```python
from build123d import *

# Parameters (mm, degrees)
CUT_EXTRUDE1_DEPTH = 46.95650117230423
FILLET1_R          = 10


with BuildPart() as part:
    # Sketch1 → Revolve1 (revolve)
    with BuildSketch(Plane.XY, mode=Mode.PRIVATE) as revolve1_sk:
        with BuildLine():
            Line((-20, 4.7625), (-20, 14.5))
            Line((-20, 14.5), (-15.328636266651278, 14.5))
            ThreePointArc((-15.328636266651278, 14.5), (1.5695766523512105, 11), (18.08622279664887, 16))
            Line((18.08622279664887, 16), (20, 16))
            Line((20, 16), (20, 4.7625))
            Line((20, 4.7625), (16.825, 4.7625))
            Line((16.825, 4.7625), (16.825, 3.96875))
            Line((16.825, 3.96875), (-16.825, 3.96875))
            Line((-16.825, 3.96875), (-16.825, 4.7625))
            Line((-16.825, 4.7625), (-20, 4.7625))
        make_face()
    revolve(revolve1_sk.sketch.rotate(Axis((-20, 0, 0), (1, 0, 0)), 90), axis=Axis((-20, 0, 0), (1, 0, 0)))

    # Sketch2 → Cut-Extrude1 (cut, through all)
    with BuildSketch(Plane(origin=(20, 0, 0), x_dir=(0, 0, -1), z_dir=(1, 0, 0))):
        Polygon((-0.9875675416844027, 5.918167820416334), (0, 8), (0.9875675416844045, 5.918167820416334), (2.5975957536374685, 7.56653793360508), (2.855684358222442, 5.276842507238936), (4.913701701517343, 6.313124075171151), (4.414343464038791, 4.06368942975445), (6.69733182610023, 4.375585264979419), (5.494639959930347, 2.4101725479178207), (7.7552021275146465, 1.9638838971263979), (5.979506958040023, 0.4954760728339973), (7.972675944053363, -0.6606347637786543), (5.8164015956359885, -1.47291292284479), (7.326186613240466, -3.2135633972237505), (5.022998869575178, -3.2816889487345575), (5.885791285385062, -5.418252573005925), (3.685276276138015, -4.7348430563783594), (3.807579144296598, -7.035790009651912), (1.948196815228109, -5.674903450203807), (1.3167567222458805, -7.890890427221779), (8.4e-15, -6), (-1.3167567222458623, -7.8908904272217795), (-1.9481968152280928, -5.674903450203809), (-3.80757914429658, -7.035790009651914), (-3.685276276137998, -4.7348430563783666), (-5.885791285385044, -5.418252573005935), (-5.022998869575163, -3.2816889487345664), (-7.326186613240452, -3.213563397223763), (-5.816401595635977, -1.4729129228448008), (-7.9726759440533534, -0.6606347637786659), (-5.979506958040015, 0.4954760728339881), (-7.75520212751464, 1.9638838971263866), (-5.4946399599303435, 2.4101725479178118), (-6.697331826100229, 4.375585264979409), (-4.41434346403879, 4.063689429754444), (-4.913701701517344, 6.313124075171145), (-2.855684358222442, 5.276842507238932), (-2.5975957536374694, 7.566537933605075), align=None)
    extrude(amount=-CUT_EXTRUDE1_DEPTH, mode=Mode.SUBTRACT)

    # Fillet1
    # the kernel refuses this fillet: 10 mm, written as the material it takes off along each edge
    with BuildSketch(Plane(origin=(18.08622279664887, 0, 0), x_dir=(0, 1.1e-16, 1), z_dir=(0, 1, -1.1e-16))) as fillet1_piece_1:
        with BuildLine():
            CenterArc((6.027123801609688, 2.6498073192975404), FILLET1_R, 332.5612146984912, 23.217826405433588)
            Line((15.999999999999996, 1.913777203351131), (16.1994575239678, 1.8990566010322034))
            ThreePointArc((16.1994575239678, 1.8990566010322034), (16.2, 0.9568886016755656), (16.199999999999996, 0))
            Line((16.199999999999996, 0), (16.17122736238995, -0.10334984455228025))
            ThreePointArc((16.17122736238995, -0.10334984455228025), (15.609829730901891, -1.0681006002986955), (15.079661114712898, -2.050359506983643))
            Line((15.079661114712898, -2.050359506983643), (14.902160383083423, -1.9581993731349918))
        make_face()
    revolve(axis=Axis((18.08622279664887, 0, 0), (1, 0, 0)), mode=Mode.SUBTRACT)
    with BuildSketch(Plane(origin=(-15.328636266651278, 0, 0), x_dir=(0, 1.1e-16, 1), z_dir=(0, 1, -1.1e-16))) as fillet1_piece_2:
        with BuildLine():
            CenterArc((4.5, -2.1548222421926884), FILLET1_R, 0, 22.862521626171226)
            Line((13.714397426275884, 1.7303907597726322), (13.898685374801401, 1.8080950198119385))
            ThreePointArc((13.898685374801401, 1.8080950198119385), (14.277562788256734, 0.9425411788785816), (14.67979879096138, 0.08759220723800709))
            Line((14.67979879096138, 0.08759220723800709), (14.7, 0))
            Line((14.7, 0), (14.7, -2.1548222421926884))
            Line((14.7, -2.1548222421926884), (14.5, -2.1548222421926884))
        make_face()
    revolve(axis=Axis((-15.328636266651278, 0, 0), (1, 0, 0)), mode=Mode.SUBTRACT)


solid = part.part
```
For this review, take the finished solid that the model builds, in its own axes (mm). Coordinates: 2 decimals unless noted, no trailing zeros. Use CSV: the item, a comma, the result in double quotes. Start each with the question number.
Item 1: Insertion check: pin 1 (1.5 mm diameter, centred on x = -10, y = -1.5, fed in from -Z); pin 2 (3 mm diameter, centred on x = 10, y = 11, fed in from -Z); pin 3 (4 mm diameter, centred on x = -2, z = -7, fed in from +Y). Each pin has a flat end and moves straight along its axis. Give the tip position at first contact, or say it passes through.
Item 2: Draft analysis for pull direction Z (two halves, no side actions). For faces 1 (the face through (20, 3, 7)), 2 (the face through (0.28, -5.07, 4.77)), 3 (the face through (-18.724, 12.864, 6.691)), state which applies: pulls with the +Z half, pulls with the -Z half, needs draft (parallel to the pull), parting line crosses it, or undercut.
Item 3: Wall thickness on probe 1 along Z at (x, y) = (0, -2.5); probe 2 along Z at (x, y) = (-2, 3.5); probe 3 along Z at (x, y) = (-1.5, 7): over which ranges is each line inside the solid? List them lowest first.
Derived:
1,pin 1,"stops at z = -12.58"
1,pin 2,"stops at z = -8.14"
1,pin 3,"stops at y = 9.83"
2,face 1,"needs draft"
2,face 2,"undercut"
2,face 3,"parting line crosses it"
3,probe 1,"z = -10.68 to -6.71, 6.71 to 10.68"
3,probe 2,"z = -10.45 to -6.16, 6.16 to 10.45"
3,probe 3,"z = -8.48 to -2.66, -2.04 to -0.47, 0.47 to 2.04, 2.66 to 8.48"
